```python
from build123d import *

# Parameters (mm, degrees)
BASEHEAD_DEPTH = 3.875
SKETCH4_W      = 0.5
SKETCH4_H      = 10.618802154


# Read off the part's stored shape, not the designer's step: HeadChamfer
with BuildPart() as part:
    # Sketch1 → BaseHead (new body)
    with BuildSketch(Plane(origin=(0, 0, 0), x_dir=(0, 0, -1), z_dir=(1, 0, 0))):
        Polygon((4, 2.309401077), (4, -2.309401077), (0, -4.618802154), (-4, -2.309401077), (-4, 2.309401077), (0, 4.618802154), align=None)
    extrude(amount=BASEHEAD_DEPTH)

    # HeadChamfer outline → HeadChamfer (revolve, cut)
    with BuildSketch(Plane.YX):
        Polygon((4.618802148, 0.357265587), (3.999999382, -3.57e-07), (4.618802154, -3.57e-07), align=None)
    revolve(axis=Axis((0, 0, 0), (1, 0, 0)), mode=Mode.SUBTRACT)

    # HeadChamfer 2 outline → HeadChamfer 2 (revolve)
    with BuildSketch(Plane.YX):
        Polygon((2.5, 3.875), (2.5, 158.43), (2.055, 158.875), (0, 158.875), (0, 3.875), align=None)
    revolve(axis=Axis((0, 0, 0), (1, 0, 0)))

    # Sketch4 → BearingFace (revolve, cut)
    with BuildSketch(Plane.XY, mode=Mode.PRIVATE) as bearingface_sk:
        with Locations((3.625, 9.309401077)):
            Rectangle(SKETCH4_W, SKETCH4_H)
    revolve(bearingface_sk.sketch.rotate(Axis((0, 0, 0), (1, 0, 0)), 90), axis=Axis((0, 0, 0), (1, 0, 0)), mode=Mode.SUBTRACT)


solid = part.part
```
Here's how the part is built. I have some questions about the finished solid (model axes, mm). A direction names the side the tool comes from. Coordinates: 2 decimals unless noted, no trailing zeros. Order: outer loops, then holes, each group sorted by start corner. A loop starts at its lowest first (then second) coordinate and runs counter-clockwise, first axis right, second up.
1) Imagine slicing it at A-A on x = 110. List the corners of the cut face in (y, z) for me.
2) Which directions (+Z, -Z, +X, -X, +Y, -Y) give clear straight access to the entire face, cutting with the end or side of a thin tool? Please do faces 1 (the face through (1.66, -3.48, 1.97)), 2 (the face through (3.628, 3.905, -0.867)).
3) I need wall thicknesses on line 1 (Z direction, x = 67, y = -0.25); line 2 (X direction, y = 3.25, z = 1.75) (3 decimals). Which ranges of each line are inside material? Lowest first, please.
4) Will these pins go through, and if not, where does the flat tip stop? pin 1 (0.9 mm diameter, centred on y = -4, z = 0, fed in from +X) (3 decimals); pin 2 (1 mm diameter, centred on x = 109, z = 2.5, fed in from -Y); pin 3 (1.6 mm diameter, centred on y = 2, z = -2.5, fed in from +X).
Response values:
1. outline: circle Ø5 at (0, 0)
2. face 1: +Z, +X, -X, -Y
2. face 2: +X
3. line 1: z = -2.49 to 2.49
3. line 2: x = 0 to 3.875
4. pin 1: stops at x = 3.875
4. pin 2: stops at y = -1.5
4. pin 3: stops at x = 158.53
